Read the model definition and answer for the solid it produces. Units are mm, in the model's axes. Coordinates: 2 decimals unless noted, no trailing zeros. Order: outer loops, then holes, each group sorted by start corner. A loop starts at its lowest first (then second) coordinate and runs counter-clockwise, first axis right, second up. Notation, with made-up numbers: (48.25, 85.25) -> (97.25, 85.25) arc R27 cw to (97.25, 109.25) -> close; hole circle Ø4 at (22, -35.75). An arc over 180 degrees is marked (long way). Answer in a Markdown table with one row per item.
from build123d import *

# Parameters (mm, degrees)
F1_DEPTH    = 76.2
F2_T1_DEPTH = 85.725
F2_T3_DEPTH = 85.1802561211


# Not quite as in the source:
# - a fillet or chamfer that OpenCascade refuses, or shapes differently, is made with other operations: its cross-section is extruded or revolved along the edge and cut away or added


with BuildPart() as f1:
    # F0 (on Top) → F1 (new body)
    with BuildSketch(Plane.XY):
        Polygon((-19.05, -3.175), (19.05, -3.175), (19.05, 3.175), (-19.05, 3.175), (-19.05, 1.905), (17.78, 1.905), (17.78, -1.905), (-19.05, -1.905), align=None)
    extrude(amount=F1_DEPTH)

    # F2: fillet of radius 1.905 on 4 edges, made by hand

    # F2_s2 → F2_t1 (cut)
    with BuildSketch(Plane.XY.offset(-4.7625)):
        with BuildLine():
            ThreePointArc((19.05, 1.27), (18.4920384182, 2.6170384182), (17.145, 3.175))
            Line((17.145, 3.175), (19.05, 3.175))
            Line((19.05, 3.175), (19.05, 1.27))
        make_face()
        with BuildLine():
            ThreePointArc((17.145, -3.175), (18.4920384182, -2.6170384182), (19.05, -1.27))
            Line((19.05, -1.27), (19.05, -3.175))
            Line((19.05, -3.175), (17.145, -3.175))
        make_face()
    extrude(amount=F2_T1_DEPTH, mode=Mode.SUBTRACT)

    # F2_s4 → F2_t3 (cut)
    with BuildSketch(Plane.XY.offset(-4.4901280605)):
        with BuildLine():
            ThreePointArc((-19.05, -1.905), (-18.3538010386, -2.8254259867), (-17.2539487758, -3.175))
            Line((-17.2539487758, -3.175), (-19.05, -3.175))
            Line((-19.05, -3.175), (-19.05, -1.905))
        make_face()
        with BuildLine():
            ThreePointArc((-17.2539487758, 3.175), (-18.3538010386, 2.8254259867), (-19.05, 1.905))
            Line((-19.05, 1.905), (-19.05, 3.175))
            Line((-19.05, 3.175), (-17.2539487758, 3.175))
        make_face()
    extrude(amount=F2_T3_DEPTH, mode=Mode.SUBTRACT)


solid = f1.part
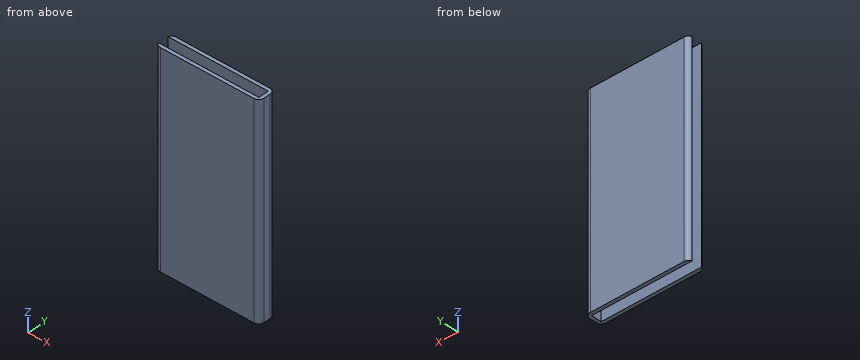
Q1. The part is cut by section A-A (x = 15). Write down the section's boundary in (y, z) (3 decimals).
Outcome:
| item | result |
|---|---|
| outline | (-3.175, 0) -> (-1.905, 0) -> (-1.905, 76.2) -> (-3.175, 76.2) -> close; (1.905, 0) -> (3.175, 0) -> (3.175, 76.2) -> (1.905, 76.2) -> close |
Q2. The part is cut by section C-C (y = -0.5). Write down the section's boundary in (x, z), then the cut area to 3 significant figures.
Outcome:
| item | result |
|---|---|
| outline | (17.78, 0) -> (19.05, 0) -> (19.05, 76.2) -> (17.78, 76.2) -> close |
| area | 96.8 mm² |
Q3. Given pin 1 (1.1 mm diameter, centred on y = -1, z = 33.5, fed in from -X), flat-ended and moving along its own axis, determine where the tip first touches the part or whether it passes through.
Outcome:
| item | result |
|---|---|
| pin 1 | x = 17.78 |
Q4. The part is cut by section B-B (z = 70.5). Write down the section's boundary in (x, y) (3 decimals).
Outcome:
| item | result |
|---|---|
| outline | (-19.05, -1.905) arc R1.905 ccw to (-17.254, -3.175) -> (17.145, -3.175) arc R1.905 ccw to (19.05, -1.27) -> (19.05, 1.27) arc R1.905 ccw to (17.145, 3.175) -> (-17.254, 3.175) arc R1.905 ccw to (-19.05, 1.905) -> (17.78, 1.905) -> (17.78, -1.905) -> close |
Q5. Consider line 1 (Y direction, x = -17, z = 29.5) (3 decimals); line 2 (X direction, y = -0.5, z = 68); line 3 (X direction, y = 2, z = 26). Determine where each line is inside the solid, lowest interval first.
Outcome:
| item | result |
|---|---|
| line 1 | -3.175 to -1.905, 1.905 to 3.175 |
| line 2 | 17.78 to 19.05 |
| line 3 | -19.01 to 18.9 |
